from build123d import *

# Parameters (mm, degrees)
SKIZZE3_R                       = 1.5
AUFSATZ_LINEAR_AUSTRAGEN1_DEPTH = 1.5


with BuildPart() as part:
    # Skizze3 → Aufsatz-Linear austragen1 (new body, symmetric)
    with BuildSketch(Plane.XY):
        Polygon((-30.75, 10), (10.75, 10), (10.75, -10), (17.75, -10), (17.75, 17), (-37.75, 17), (-37.75, -10), (-30.75, -10), align=None)
        with Locations((-34.25, 5)):
            Circle(SKIZZE3_R, mode=Mode.SUBTRACT)
        with Locations((-34.25, -5)):
            Circle(SKIZZE3_R, mode=Mode.SUBTRACT)
        with Locations((14.25, 5)):
            Circle(SKIZZE3_R, mode=Mode.SUBTRACT)
        with Locations((14.25, -5)):
            Circle(SKIZZE3_R, mode=Mode.SUBTRACT)
    extrude(amount=AUFSATZ_LINEAR_AUSTRAGEN1_DEPTH, both=True)


solid = part.part
Geometry: final body of the model. Coordinates: model frame, mm. A direction names the side the tool comes from. Round coordinates to 2 decimals unless told otherwise and drop trailing zeros. Order: outer loops, then holes, each group sorted by start corner. A loop starts at its lowest first (then second) coordinate and runs counter-clockwise, first axis right, second up. Notation, with made-up numbers: (-4, 49.5) -> (39, 49.5) arc R21 cw to (39, 79.5) -> close; hole circle Ø2 at (81.5, 25.5). An arc over 180 degrees is marked (long way). Put each result on its own line as item: value. Start each with the question number.
Q1. Section D-D on x = -16.5. Return the cut outline in (y, z), and give its area (3 significant figures).
Q2. Section A-A on x = 14.25. Return the cut outline in (y, z), and give its area (3 significant figures).
Q3. Section C-C on z = 0.65. Return the cut outline in (x, y), and give its area (3 significant figures).
Q4. Pull-direction query (Y, two-part tool) for faces 1 (the flat face through (14, -10, 0)), 2 (the flat face through (-37.75, 4, 0)), 3 (the cylindrical face through (-35.44, 4.09, -0.02)); classes: +Y half, -Y half, draft (parallel to the pull), parting line (faces both ways), or undercut.
Q5. Line query: probe 1 along Y at (x, z) = (14.25, -0.2); probe 2 along X at (y, z) = (-6.25, -0.1); probe 3 along X at (y, z) = (0.75, -1). Output: solid intervals per line, ascending.
Q6. First-contact query: pin 1 (0.9 mm diameter, centred on x = -9, z = -0.5, fed in from -Y); pin 2 (4 mm diameter, centred on x = -34.25, y = 5, fed in from -Z). Flat tips, straight axial feed; report the tip coordinate or a pass-through.
Q7. Reachability of faces 4 (the flat face through (10.75, 0, 0)), 5 (the cylindrical face through (-35.44, -5.91, -0.02)) from +Z, -Z, +X, -X, +Y, -Y: full face, straight path, thin tool, end or side. Return the list, or none.
Q8. Section B-B on y = -5. Return the cut outline in (x, z).
Ans:
1. outline: (10, -1.5) -> (17, -1.5) -> (17, 1.5) -> (10, 1.5) -> close
1. area: 21.0 mm2
2. outline: (-10, -1.5) -> (-6.5, -1.5) -> (-6.5, 1.5) -> (-10, 1.5) -> close; (-3.5, -1.5) -> (3.5, -1.5) -> (3.5, 1.5) -> (-3.5, 1.5) -> close; (6.5, -1.5) -> (17, -1.5) -> (17, 1.5) -> (6.5, 1.5) -> close
2. area: 63.0 mm2
3. outline: (-37.75, -10) -> (-30.75, -10) -> (-30.75, 10) -> (10.75, 10) -> (10.75, -10) -> (17.75, -10) -> (17.75, 17) -> (-37.75, 17) -> close; hole circle Ø3 at (-34.25, -5); hole circle Ø3 at (-34.25, 5); hole circle Ø3 at (14.25, -5); hole circle Ø3 at (14.25, 5)
3. area: 640 mm2
4. face 1: -Y half
4. face 2: draft
4. face 3: undercut
5. probe 1: y = -10 to -6.5, -3.5 to 3.5, 6.5 to 17
5. probe 2: x = -37.75 to -35.08, -33.42 to -30.75, 10.75 to 13.42, 15.08 to 17.75
5. probe 3: x = -37.75 to -30.75, 10.75 to 17.75
6. pin 1: stops at y = 10
6. pin 2: stops at z = -1.5
7. face 4: +Z, -Z, -Y
7. face 5: +Z, -Z
8. outline: (-37.75, -1.5) -> (-35.75, -1.5) -> (-35.75, 1.5) -> (-37.75, 1.5) -> close; (-32.75, -1.5) -> (-30.75, -1.5) -> (-30.75, 1.5) -> (-32.75, 1.5) -> close; (10.75, -1.5) -> (12.75, -1.5) -> (12.75, 1.5) -> (10.75, 1.5) -> close; (15.75, -1.5) -> (17.75, -1.5) -> (17.75, 1.5) -> (15.75, 1.5) -> close
